Part model, mm, in its own coordinate system. A direction names the side the tool comes from. Round coordinates to 2 decimals unless told otherwise and drop trailing zeros. Loops run counter-clockwise (first coordinate to the right, second up) from the corner with the lowest first, then second, coordinate; pieces in that order, holes last.
(1) Flat gauge pins, fed straight in: pin 1 (8 mm diameter, centred on x = 20, z = -28.5, fed in from -Y); pin 2 (2 mm diameter, centred on x = 17, z = -11.5, fed in from +Y); pin 3 (1 mm diameter, centred on x = 32.5, y = -29.5, fed in from -Z). Where does each tip first touch, or does it go through?
(2) Cut at C-C on y = -84.5. Count the separate pieces of the cut face and the enclosed holes in it, then the cut area to 3 significant figures.
(3) Cut at B-B on z = -52. List the corners of the cut face in (x, y), then the cut area to 3 significant figures.
(4) Probe probe 1 along Z at (x, y) = (35, -91); probe 2 along Y at (x, z) = (15, -8); probe 3 along Z at (x, y) = (19, -89.5). List the from-to ranges inside material, lowest first.
(5) Mould opens along Y. For faces 1 (the face through (19.72, -0.762, -9.339)), 2 (the face through (19.72, -99.238, -90.661)), 3 (the face through (19.72, -91.344, -2.645)) say: +Y half, -Y half, draft (parallel to the pull), parting line (faces both ways), or undercut.
(6) Cut at A-A on y = -43. List the corners of the cut face in (x, z), then the cut area to 3 significant figures.
(7) Tool access for faces 4 (the face through (19.72, -49.831, -20.013)), 5 (the face through (19.72, -99.194, -9.442)), 6 (the face through (19.72, -9.339, -99.238)), 7 (the face through (19.72, -0.806, -90.558)): list every direction of +Z, -Z, +X, -X, +Y, -Y with a clear straight run to the whole face (end or side of a thin tool).
from build123d import *

# Parameters (mm, degrees)
BOSS_EXTRUDE1_DEPTH = 40
FILLET1_R           = 2


with BuildPart() as part:
    # Sketch1 → Boss-Extrude1 (new body)
    with BuildSketch(Plane(origin=(0, 0, 0), x_dir=(0, 0, -1), z_dir=(1, 0, 0))):
        with BuildLine():
            Line((100, 0), (100, -5.509803926))
            ThreePointArc((100, -5.509803926), (99.216139085, -9.390883719), (96.987443928, -12.663518161))
            add(Edge.make_bspline(
                [(96.987443928, -12.663518161), (94.284956793, -15.303192699), (88.725985213, -22.501160026), (85.001584131, -31.833431523), (83.50630434, -37.738521084), (83.320771704, -38.525392743)],
                knots=[0.087567714, 0.087567714, 0.087567714, 0.087567714, 0.336049895, 0.688961666, 0.74236025, 0.74236025, 0.74236025, 0.74236025], degree=3))
            ThreePointArc((83.320771704, -38.525392743), (81.98629737, -50), (83.320771704, -61.474607257))
            add(Edge.make_bspline(
                [(96.987443928, -87.336481839), (94.284956793, -84.696807301), (88.725985213, -77.498839974), (85.001584131, -68.166568477), (83.50630434, -62.261478916), (83.320771704, -61.474607257)],
                knots=[0.087567714, 0.087567714, 0.087567714, 0.087567714, 0.336049895, 0.688961666, 0.74236025, 0.74236025, 0.74236025, 0.74236025], degree=3))
            ThreePointArc((96.987443928, -87.336481839), (99.216139085, -90.609116281), (100, -94.490196074))
            Line((100, -94.490196074), (100, -100))
            Line((100, -100), (94.490196074, -100))
            ThreePointArc((94.490196074, -100), (90.609116281, -99.216139085), (87.336481839, -96.987443928))
            add(Edge.make_bspline(
                [(87.336481839, -96.987443928), (84.696807301, -94.284956793), (77.498839974, -88.725985213), (68.166568477, -85.001584131), (62.261478916, -83.50630434), (61.474607257, -83.320771704)],
                knots=[0.087567714, 0.087567714, 0.087567714, 0.087567714, 0.336049895, 0.688961666, 0.74236025, 0.74236025, 0.74236025, 0.74236025], degree=3))
            ThreePointArc((61.474607257, -83.320771704), (50, -81.98629737), (38.525392743, -83.320771704))
            add(Edge.make_bspline(
                [(12.663518161, -96.987443928), (15.303192699, -94.284956793), (22.501160026, -88.725985213), (31.833431523, -85.001584131), (37.738521084, -83.50630434), (38.525392743, -83.320771704)],
                knots=[0.087567714, 0.087567714, 0.087567714, 0.087567714, 0.336049895, 0.688961666, 0.74236025, 0.74236025, 0.74236025, 0.74236025], degree=3))
            ThreePointArc((12.663518161, -96.987443928), (9.390883719, -99.216139085), (5.509803926, -100))
            Line((5.509803926, -100), (0, -100))
            Line((0, -100), (0, -94.490196074))
            ThreePointArc((0, -94.490196074), (0.783860915, -90.609116281), (3.012556072, -87.336481839))
            add(Edge.make_bspline(
                [(3.012556072, -87.336481839), (5.715043207, -84.696807301), (11.274014787, -77.498839974), (14.998415869, -68.166568477), (16.49369566, -62.261478916), (16.679228296, -61.474607257)],
                knots=[0.087567714, 0.087567714, 0.087567714, 0.087567714, 0.336049895, 0.688961666, 0.74236025, 0.74236025, 0.74236025, 0.74236025], degree=3))
            ThreePointArc((16.679228296, -61.474607257), (18.01370263, -50), (16.679228296, -38.525392743))
            add(Edge.make_bspline(
                [(3.012556072, -12.663518161), (5.715043207, -15.303192699), (11.274014787, -22.501160026), (14.998415869, -31.833431523), (16.49369566, -37.738521084), (16.679228296, -38.525392743)],
                knots=[0.087567714, 0.087567714, 0.087567714, 0.087567714, 0.336049895, 0.688961666, 0.74236025, 0.74236025, 0.74236025, 0.74236025], degree=3))
            ThreePointArc((3.012556072, -12.663518161), (0.783860915, -9.390883719), (0, -5.509803926))
            Line((0, -5.509803926), (0, 0))
            Line((0, 0), (5.509803926, 0))
            ThreePointArc((5.509803926, 0), (9.390883719, -0.783860915), (12.663518161, -3.012556072))
            add(Edge.make_bspline(
                [(12.663518161, -3.012556072), (15.303192699, -5.715043207), (22.501160026, -11.274014787), (31.833431523, -14.998415869), (37.738521084, -16.49369566), (38.525392743, -16.679228296)],
                knots=[0.087567714, 0.087567714, 0.087567714, 0.087567714, 0.336049895, 0.688961666, 0.74236025, 0.74236025, 0.74236025, 0.74236025], degree=3))
            ThreePointArc((38.525392743, -16.679228296), (50, -18.01370263), (61.474607257, -16.679228296))
            add(Edge.make_bspline(
                [(87.336481839, -3.012556072), (84.696807301, -5.715043207), (77.498839974, -11.274014787), (68.166568477, -14.998415869), (62.261478916, -16.49369566), (61.474607257, -16.679228296)],
                knots=[0.087567714, 0.087567714, 0.087567714, 0.087567714, 0.336049895, 0.688961666, 0.74236025, 0.74236025, 0.74236025, 0.74236025], degree=3))
            ThreePointArc((87.336481839, -3.012556072), (90.609116281, -0.783860915), (94.490196074, 0))
            Line((94.490196074, 0), (100, 0))
        make_face()
        with BuildLine():
            Line((2, -2), (2, -5.509803926))
            ThreePointArc((2, -5.509803926), (2.627088732, -8.61466776), (4.410044858, -11.232775314))
            add(Edge.make_bspline(
                [(4.410044858, -11.232775314), (5.338828529, -12.139971717), (7.119384177, -14.045499285), (10.298925927, -18.104117855), (13.619253938, -23.620299694), (16.6302594, -30.724007948), (18.043201909, -35.595313625), (18.625849322, -38.066408453)],
                knots=[0.087567714, 0.087567714, 0.087567714, 0.087567714, 0.169416781, 0.251265848, 0.414963982, 0.578662116, 0.74236025, 0.74236025, 0.74236025, 0.74236025], degree=3))
            ThreePointArc((18.625849322, -38.066408453), (20.01370263, -50), (18.625849322, -61.933591547))
            add(Edge.make_bspline(
                [(18.625849322, -61.933591547), (18.043201909, -64.404686375), (16.6302594, -69.275992052), (13.619253938, -76.379700306), (10.298925927, -81.895882145), (7.119384178, -85.954500715), (5.338828529, -87.860028283), (4.410044858, -88.767224686)],
                knots=[0.087567714, 0.087567714, 0.087567714, 0.087567714, 0.251265848, 0.414963982, 0.578662116, 0.660511183, 0.74236025, 0.74236025, 0.74236025, 0.74236025], degree=3))
            ThreePointArc((4.410044858, -88.767224686), (2.627088732, -91.38533224), (2, -94.490196074))
            Line((2, -94.490196074), (2, -98))
            Line((2, -98), (5.509803926, -98))
            ThreePointArc((5.509803926, -98), (8.61466776, -97.372911268), (11.232775314, -95.589955142))
            add(Edge.make_bspline(
                [(11.232775314, -95.589955142), (12.139971717, -94.661171471), (14.045499285, -92.880615823), (18.104117855, -89.701074073), (23.620299694, -86.380746062), (30.724007948, -83.3697406), (35.595313625, -81.956798091), (38.066408453, -81.374150678)],
                knots=[0.087567714, 0.087567714, 0.087567714, 0.087567714, 0.169416781, 0.251265848, 0.414963982, 0.578662116, 0.74236025, 0.74236025, 0.74236025, 0.74236025], degree=3))
            ThreePointArc((38.066408453, -81.374150678), (50, -79.98629737), (61.933591547, -81.374150678))
            add(Edge.make_bspline(
                [(61.933591547, -81.374150678), (64.404686375, -81.956798091), (69.275992052, -83.3697406), (76.379700306, -86.380746062), (81.895882145, -89.701074073), (85.954500715, -92.880615823), (87.860028283, -94.661171471), (88.767224686, -95.589955142)],
                knots=[0.087567714, 0.087567714, 0.087567714, 0.087567714, 0.251265848, 0.414963982, 0.578662116, 0.660511183, 0.74236025, 0.74236025, 0.74236025, 0.74236025], degree=3))
            ThreePointArc((88.767224686, -95.589955142), (91.38533224, -97.372911268), (94.490196074, -98))
            Line((94.490196074, -98), (98, -98))
            Line((98, -98), (98, -94.490196074))
            ThreePointArc((98, -94.490196074), (97.372911268, -91.38533224), (95.589955142, -88.767224686))
            add(Edge.make_bspline(
                [(95.589955142, -88.767224686), (94.661171471, -87.860028283), (92.880615823, -85.954500715), (89.701074073, -81.895882145), (86.380746062, -76.379700306), (83.3697406, -69.275992052), (81.956798091, -64.404686375), (81.374150678, -61.933591547)],
                knots=[0.087567714, 0.087567714, 0.087567714, 0.087567714, 0.169416781, 0.251265848, 0.414963982, 0.578662116, 0.74236025, 0.74236025, 0.74236025, 0.74236025], degree=3))
            ThreePointArc((81.374150678, -61.933591547), (79.98629737, -50), (81.374150678, -38.066408453))
            add(Edge.make_bspline(
                [(81.374150678, -38.066408453), (81.956798091, -35.595313625), (83.3697406, -30.724007948), (86.380746062, -23.620299694), (89.701074073, -18.104117855), (92.880615823, -14.045499285), (94.661171471, -12.139971717), (95.589955142, -11.232775314)],
                knots=[0.087567714, 0.087567714, 0.087567714, 0.087567714, 0.251265848, 0.414963982, 0.578662116, 0.660511183, 0.74236025, 0.74236025, 0.74236025, 0.74236025], degree=3))
            ThreePointArc((95.589955142, -11.232775314), (97.372911268, -8.61466776), (98, -5.509803926))
            Line((98, -5.509803926), (98, -2))
            Line((98, -2), (94.490196074, -2))
            ThreePointArc((94.490196074, -2), (91.38533224, -2.627088732), (88.767224686, -4.410044858))
            add(Edge.make_bspline(
                [(88.767224686, -4.410044858), (87.860028283, -5.338828529), (85.954500715, -7.119384177), (81.895882145, -10.298925927), (76.379700306, -13.619253938), (69.275992052, -16.6302594), (64.404686375, -18.043201909), (61.933591547, -18.625849322)],
                knots=[0.087567714, 0.087567714, 0.087567714, 0.087567714, 0.169416781, 0.251265848, 0.414963982, 0.578662116, 0.74236025, 0.74236025, 0.74236025, 0.74236025], degree=3))
            ThreePointArc((61.933591547, -18.625849322), (50, -20.01370263), (38.066408453, -18.625849322))
            add(Edge.make_bspline(
                [(38.066408453, -18.625849322), (35.595313625, -18.043201909), (30.724007948, -16.6302594), (23.620299694, -13.619253938), (18.104117855, -10.298925927), (14.045499285, -7.119384177), (12.139971717, -5.338828529), (11.232775314, -4.410044858)],
                knots=[0.087567714, 0.087567714, 0.087567714, 0.087567714, 0.251265848, 0.414963982, 0.578662116, 0.660511183, 0.74236025, 0.74236025, 0.74236025, 0.74236025], degree=3))
            ThreePointArc((11.232775314, -4.410044858), (8.61466776, -2.627088732), (5.509803926, -2))
            Line((5.509803926, -2), (2, -2))
        make_face(mode=Mode.SUBTRACT)
    extrude(amount=BOSS_EXTRUDE1_DEPTH)

    # Fillet1
    fillet1_edges = [part.edges().sort_by_distance(p)[0] for p in [
        (20, 0, 0),
        (20, 0, -100),
        (20, -100, -100),
        (20, -100, 0),
        (20, -2, -2),
        (20, -98, -2),
        (20, -98, -98),
        (20, -2, -98),
    ]]
    fillet(fillet1_edges, radius=FILLET1_R)


solid = part.part
Final values:
1. pin 1: stops at y = -88.38
1. pin 2: stops at y = -1.33
1. pin 3: stops at z = -86.33
2. separate pieces: 4
2. enclosed holes: 0
2. area: 685 mm2
3. outline: (0, -82.03) - (40, -82.03) - (40, -80.02) - (0, -80.02) - close; (0, -19.98) - (40, -19.98) - (40, -17.97) - (0, -17.97) - close
3. area: 160 mm2
4. probe 1: z = -99.37 to -97.2, -83.51 to -80.02, -19.98 to -16.49, -2.8 to -0.63
4. probe 2: y = -99.68 to -97.6, -84.8 to -81.48, -18.52 to -15.2, -2.4 to -0.32
4. probe 3: z = -98.67 to -96.25, -81.38 to -77.57, -22.43 to -18.62, -3.75 to -1.33
5. face 1: +Y half
5. face 2: -Y half
5. face 3: undercut
6. outline: (0, -82.48) - (40, -82.48) - (40, -80.46) - (0, -80.46) - close; (0, -19.54) - (40, -19.54) - (40, -17.52) - (0, -17.52) - close
6. area: 162 mm2
7. face 4: +X, -X
7. face 5: +X, -X, -Y
7. face 6: -Z, +X, -X
7. face 7: +X, -X, +Y
